```python
from build123d import *

# Parameters (mm, degrees)
PAD_DEPTH       = 7
PAD001_DEPTH    = 2
FILLET_R        = 20
FILLET001_R     = 20
FILLET002_R     = 1
FILLET003_R     = 1
POCKET_DEPTH    = 6
POCKET001_DEPTH = 5
POCKET002_DEPTH = 5


with BuildPart() as part:
    # Sketch003 → Pad (new body)
    with BuildSketch(Plane.XY.offset(69)):
        with BuildLine():
            Line((0.013913, 21), (46.663841, 21))
            ThreePointArc((46.663841, 0), (62.854257, 10.5), (46.663841, 21))
            Line((46.663841, 0), (0.013913, 0))
            Line((0.013913, 0), (0.013913, 21))
        make_face()
    extrude(amount=PAD_DEPTH)

    # Sketch → Pad001 (new body)
    with BuildSketch(Plane(origin=(0, 0, 69), x_dir=(1, 0, 0), z_dir=(0, 0, -1))):
        with BuildLine():
            Line((1.511721, -19.526379), (48.404155, -19.526379))
            ThreePointArc((48.404155, -19.526379), (60.840174, -10.38315), (48.198543, -1.526379))
            Line((1.511721, -1.526379), (48.198543, -1.526379))
            Line((1.511721, -1.526379), (1.511721, -19.526379))
        make_face()
    extrude(amount=PAD001_DEPTH)

    # Fillet
    fillet_edges = [part.edges().sort_by_distance(p)[0] for p in [
        (46.663841, 21, 72.5),
    ]]
    fillet(fillet_edges, radius=FILLET_R)

    # Fillet001
    fillet001_edges = [part.edges().sort_by_distance(p)[0] for p in [
        (46.663841, 0, 72.5),
    ]]
    fillet(fillet001_edges, radius=FILLET001_R)

    # Fillet002
    fillet002_edges = [part.edges().sort_by_distance(p)[0] for p in [
        (0.013913, 0, 72.5),
    ]]
    fillet(fillet002_edges, radius=FILLET002_R)

    # Fillet003
    fillet003_edges = [part.edges().sort_by_distance(p)[0] for p in [
        (0.013913, 21, 72.5),
    ]]
    fillet(fillet003_edges, radius=FILLET003_R)

    # Sketch004 → Pocket (cut)
    with BuildSketch(Plane.XY.offset(76)):
        with BuildLine():
            Line((1.482056, 1.60733), (47.999464, 1.60733))
            ThreePointArc((47.999464, 1.60733), (60.81663, 10.193947), (48.593783, 19.60733))
            Line((1.482056, 19.60733), (48.593783, 19.60733))
            Line((1.482056, 19.60733), (1.482056, 1.60733))
        make_face()
    extrude(amount=-POCKET_DEPTH, mode=Mode.SUBTRACT)

    # Sketch005 → Pocket001 (cut)
    with BuildSketch(Plane(origin=(0.013913, 0, 69), x_dir=(0, -1, 0), z_dir=(-1, 0, 0))):
        with BuildLine():
            ThreePointArc((-16.232645, 5.858135), (-17.922069, 4.168711), (-16.232645, 2.479286))
            Line((-16.232645, 2.479286), (-4.73362, 2.479286))
            ThreePointArc((-4.73362, 2.479286), (-3.044195, 4.168711), (-4.73362, 5.858135))
            Line((-16.232645, 5.858135), (-4.73362, 5.858135))
        make_face()
    extrude(amount=-POCKET001_DEPTH, mode=Mode.SUBTRACT)

    # Sketch006 → Pocket002 (cut)
    with BuildSketch(Plane.XY.offset(70)):
        with BuildLine():
            ThreePointArc((32.291425, 16.37623), (30.46347, 18.204185), (28.635515, 16.37623))
            Line((28.635515, 16.37623), (28.635515, 4.934208))
            ThreePointArc((28.635515, 4.934208), (30.46347, 3.106253), (32.291425, 4.934208))
            Line((32.291425, 16.37623), (32.291425, 4.934208))
        make_face()
    extrude(amount=-POCKET002_DEPTH, mode=Mode.SUBTRACT)


solid = part.part
```
Geometry check sheet. Reference: the model listing, model coordinates, mm. A direction names the side the tool comes from. Round coordinates to 2 decimals unless told otherwise and drop trailing zeros. Write each loop counter-clockwise with the first axis right and the second up, starting at its lowest first coordinate (ties: lowest second). Pieces come first, ordered by that corner, then holes. Notation, with made-up numbers: (-33.75, 85.5) - (4.25, 85.5) arc R24 ccw to (4.25, 95.5) - close; hole circle Ø6 at (87, 0). An arc over 180 degrees is marked (long way). Write each question's results on one line, items separated by ' | '.
(1) Thickness scan on probe 1 along Y at (x, z) = (33, 71.25); probe 2 along Z at (x, y) = (47, 16.5); probe 3 along Y at (x, z) = (46, 74.75). Record the ranges inside material, lowest first. Write a range as from..to.
Computed:
probe 1: y = 0..1.61, 19.61..21 | probe 2: z = 67..70 | probe 3: y = -0.16..1.61, 19.61..21.16
(2) Sectioned sample at A-A, the plane y = 10.5. Enter the section's corners in (x, z), plus the area to 3 significant figures.
Computed:
outline: (0.01, 69) - (1.51, 69) - (1.51, 67) - (28.64, 67) - (28.64, 70) - (1.48, 70) - (1.48, 71.48) - (0.01, 71.48) - close; (0.01, 74.86) - (1.48, 74.86) - (1.48, 76) - (0.01, 76) - close; (32.29, 67) - (60.84, 67) - (60.84, 69) - (62.85, 69) - (62.85, 76) - (60.82, 76) - (60.82, 70) - (32.29, 70) - close | area: 187 mm^2
(3) Sectioned sample at B-B, the plane x = 21. Enter the section's corners in (y, z).
Computed:
outline: (0, 69) - (1.53, 69) - (1.53, 67) - (19.53, 67) - (19.53, 69) - (21, 69) - (21, 76) - (19.61, 76) - (19.61, 70) - (1.61, 70) - (1.61, 76) - (0, 76) - close
(4) Sectioned sample at C-C, the plane z = 74. Enter the section's corners in (x, y), plus the area to 3 significant figures.
Computed:
outline: (0.01, 1) arc R1 ccw to (1.01, 0) - (43.48, 0) arc R20 cw to (48.48, -0.63) arc R11.5 ccw (long way) to (48.48, 21.63) arc R20 cw to (43.48, 21) - (1.01, 21) arc R1 ccw to (0.01, 20) - (0.01, 17.7) - (1.48, 17.7) - (1.48, 19.61) - (48.59, 19.61) arc R9.5 cw (long way) to (48, 1.61) - (1.48, 1.61) - (1.48, 3.26) - (0.01, 3.26) - close | area: 230 mm^2
(5) Set-up check for faces 4 (the face through (32.291, 11, 69)), 5 (the face through (0.74, 17.92, 73.21)), 6 (the face through (24, 11, 70)): record each of +Z, -Z, +X, -X, +Y, -Y from which the full face is reachable in a straight line by a thin tool's end or side.
Computed:
face 4: +Z, -Z | face 5: -X | face 6: +Z
(6) Depth check by flat-ended pin: pin 1 Ø1 at (y, z) = (15, 69) entering from +X; pin 2 Ø1.6 at (y, z) = (13, 67.5) entering from -X; pin 3 Ø0.6 at (x, z) = (34.5, 68) entering from -Y. Enter the tip coordinate at first touch or a pass-through.
Computed:
pin 1: stops at x = 62.14 | pin 2: stops at x = 1.51 | pin 3: stops at y = 1.53
(7) Draft check along Y on faces 1 (the face through (1, 11, 71.479)), 2 (the face through (62.85, 10.21, 72.45)), 3 (the face through (45.965, 21.155, 72.549)). Enter one of: pulls with the +Y half, pulls with the -Y half, needs draft (parallel to the pull), parting line crosses it, or undercut.
Computed:
face 1: undercut | face 2: parting line crosses it | face 3: pulls with the +Y half
(8) Sectioned sample at D-D, the plane y = 5.5. Enter the section's corners in (x, z).
Computed:
outline: (0.01, 69) - (1.51, 69) - (1.51, 67) - (28.64, 67) - (28.64, 70) - (1.48, 70) - (1.48, 71.48) - (0.01, 71.48) - close; (0.01, 74.86) - (1.48, 74.86) - (1.48, 76) - (0.01, 76) - close; (32.29, 67) - (59.42, 67) - (59.42, 69) - (61.71, 69) - (61.71, 76) - (59.39, 76) - (59.39, 70) - (32.29, 70) - close
